The model under review builds one solid part; all positions refer to its coordinate system, in mm. A direction names the side the tool comes from. Give positions to 0.01 mm unless a question says otherwise; leave off trailing zeros. Order: outer loops, then holes, each group sorted by start corner. A loop starts at its lowest first (then second) coordinate and runs counter-clockwise, first axis right, second up. Notation, with made-up numbers: (64, 1) - (116, 1) arc R15 ccw to (116, 24) - close; hole circle Ø3 at (-37, 24). An arc over 180 degrees is marked (long way). Use CSV: the item, a comma, the result in double quotes.
```python
from build123d import *

# Parameters (mm, degrees)
SKETCH2_W          = 9
SKETCH2_H          = 3
SKETCH7_R          = 2
CUT_EXTRUDE1_DEPTH = 10
SKETCH8_R          = 2
CUT_EXTRUDE2_DEPTH = 10


with BuildPart() as part:
    # Sweep1: sweep along a path in Sketch1
    with BuildLine(Plane.XY) as sweep1_path:
        Line((0, 0), (-7.5, 0))
        ThreePointArc((-7.5, 0), (-7.853553391, 0.146446609), (-8, 0.5))
        Line((-8, 0.5), (-8, 25.5))
        ThreePointArc((-8, 25.5), (-7.853553391, 25.853553391), (-7.5, 26))
        Line((-7.5, 26), (3, 26))
    # Sketch2 → Sweep1 (sweep)
    with BuildSketch(Plane(origin=(0, 0, 0), x_dir=(0, 0, -1), z_dir=(1, 0, 0))):
        with Locations((0, -1.5)):
            Rectangle(SKETCH2_W, SKETCH2_H)
    sweep(path=sweep1_path.line)

    # Sketch7 → Cut-Extrude1 (cut)
    with BuildSketch(Plane(origin=(0, 29, 0), x_dir=(1, 0, 0), z_dir=(0, 1, 0))):
        with Locations(Location((-2, 0, 0), (0, 0, 180))):
            Circle(SKETCH7_R)
    extrude(amount=-CUT_EXTRUDE1_DEPTH, mode=Mode.SUBTRACT)

    # Sketch8 → Cut-Extrude2 (cut)
    with BuildSketch(Plane(origin=(0, -3, 0), x_dir=(-1, 0, 0), z_dir=(0, -1, 0))):
        with Locations(Location((3.5, 0, 0), (0, 0, 90))):
            Circle(SKETCH8_R)
    extrude(amount=-CUT_EXTRUDE2_DEPTH, mode=Mode.SUBTRACT)


solid = part.part
```
Item 1: Tool access review of faces 5 (the face through (-10, 27.95, -0.06)), 6 (the face through (0, -2, 0)), 7 (the face through (-5.5, 0, -1.1)): name each direction out of +Z, -Z, +X, -X, +Y, -Y from which nothing blocks a thin tool from reaching the whole face with its end or side.
Results list:
face 5,"+Z, -Z, -X, +Y"
face 6,"+Z, -Z, +X, -Y"
face 7,"+Z, -Z, +X"
Item 2: Wall thickness on L1, parallel to Y at x = -4, z = 4; L2, parallel to Z at x = -2, y = 27.85; L3, parallel to X at y = 22, z = 2.25: over which ranges is each line inside the solid? List them lowest first.
Results list:
L1,"y = -3 to 0, 26 to 29"
L2,"z = -4.5 to -2, 2 to 4.5"
L3,"x = -11 to -8"
Item 3: Take a section at B-B, the plane z = -3. Give the boundary of the cut face in (x, y).
Results list:
outline,"(-11, 0.5) arc R3.5 ccw to (-7.5, -3) - (0, -3) - (0, 0) - (-7.5, 0) arc R0.5 cw to (-8, 0.5) - (-8, 25.5) arc R0.5 cw to (-7.5, 26) - (3, 26) - (3, 29) - (-7.5, 29) arc R3.5 ccw to (-11, 25.5) - close"
Item 4: Take a section at D-D, the plane x = -0.5. Give the boundary of the cut face in (y, z).
Results list:
outline,"(-3, -4.5) - (0, -4.5) - (0, 4.5) - (-3, 4.5) - close; (26, -4.5) - (29, -4.5) - (29, -1.32) - (26, -1.32) - close; (26, 1.32) - (29, 1.32) - (29, 4.5) - (26, 4.5) - close"
Item 5: Clearance check with flat-ended pins moving along their axes: pin 1 (4.5 mm diameter, centred on y = 19, z = -1.5, fed in from +X); pin 2 (1.5 mm diameter, centred on y = -1.5, z = 0, fed in from +X). State where each tip first meets the part, or that it passes through.
Results list:
pin 1,"stops at x = -8"
pin 2,"stops at x = 0"
Item 6: Take a section at A-A, the plane z = 0. Give the boundary of the cut face in (x, y), and give its area (3 significant figures).
Results list:
outline,"(-11, 0.5) arc R3.5 ccw to (-7.5, -3) - (-5.5, -3) - (-5.5, 0) - (-7.5, 0) arc R0.5 cw to (-8, 0.5) - (-8, 25.5) arc R0.5 cw to (-7.5, 26) - (-4, 26) - (-4, 29) - (-7.5, 29) arc R3.5 ccw to (-11, 25.5) - close; (-1.5, -3) - (0, -3) - (0, 0) - (-1.5, 0) - close; (0, 26) - (3, 26) - (3, 29) - (0, 29) - close"
area,"124 mm2"
Item 7: Take a section at C-C, the plane x = -3.5. Give the boundary of the cut face in (y, z).
Results list:
outline,"(-3, -4.5) - (0, -4.5) - (0, -2) - (-3, -2) - close; (-3, 2) - (0, 2) - (0, 4.5) - (-3, 4.5) - close; (26, -4.5) - (29, -4.5) - (29, -1.32) - (26, -1.32) - close; (26, 1.32) - (29, 1.32) - (29, 4.5) - (26, 4.5) - close"
Item 8: Mouldability with a two-part tool opening along Z and no side actions: class faces 1 (the face through (-8, 13, 0)), 2 (the face through (-9, 13, 4.5)), 3 (the face through (-4.7, -1.5, 1.6)), 4 (the face through (-2, 28, -2)) as pulls with the +Z half, pulls with the -Z half, needs draft (parallel to the pull), parting line crosses it, or undercut.
Results list:
face 1,"needs draft"
face 2,"pulls with the +Z half"
face 3,"undercut"
face 4,"undercut"
